Read the model definition and answer for the solid it produces. Units are mm, in the model's axes. A direction names the side the tool comes from. Coordinates: 2 decimals unless noted, no trailing zeros. Write each loop counter-clockwise with the first axis right and the second up, starting at its lowest first coordinate (ties: lowest second). Pieces come first, ordered by that corner, then holes. Notation, with made-up numbers: (29.5, 67) -> (82.5, 67) arc R30 cw to (82.5, 100) -> close; hole circle Ø3 at (32.25, 51). An arc over 180 degrees is marked (long way). One line per item, written item: value. Start each with the question number.
Autodesk Inventor part; units mm, degrees
ref_plane "YZ Plane" through (0, 0, 0) normal (1, 0, 0) x (0, 1, 0)
ref_plane "XZ Plane" through (0, 0, 0) normal (0, 1, 0) x (-1, 0, 0)
ref_plane "XY Plane" through (0, 0, 0) normal (0, 0, 1) x (1, 0, 0)
sketch "Sketch1" plane through (0, 0, 0) normal (0, 1, 0) x (-1, 0, 0)
  circle A0 centre (0, 0) radius 0.465
  dimension "d0" = 0.93
extrude "Extrusion1" add sketch "Sketch1" along normal blind 1.43
sketch "Sketch2" plane through (0, 1.43, 0) normal (0, 1, 0) x (1, 0, 0)
  circle A0 centre (0, 0) radius 0.465
  circle A1 centre (0, 0) radius 0.9625
  line L0 (0, 0) -> (7, 0)
  circle A2 centre (7, 0) radius 0.9625
  line L1 (0, -0.9625) -> (7, -0.9625)
  line L2 (0, 0.9625) -> (7, 0.9625)
  circle A3 centre (7, 0) radius 0.465
  circle A4 centre (5.02, 0) radius 0.465
  circle A5 centre (3.04, 0) radius 0.465
  dimension "d3" = 1.925
  dimension "d4" = 7
  dimension "d5" = 1.925
  dimension "d6" = 0.93
  dimension "d9" = 1.98
extrude "Extrusion2" add sketch "Sketch2" along normal blind 1.43 contours A0 | A1 | A1 L2 A2 L0 A4 A5 | L0 A5 A4 A2 L1 A1 | A2
properties part number "Servo Horn Extension"
1. A cutting plane is placed at C-C on z = 0. Give the vertices of the cut face in (x, y) (1 decimal), then the cut area to 3 significant figures.
2. A cutting plane is placed at D-D on x = 7.25. Give the vertices of the cut face in (y, z).
3. A tool of negligible diameter and unlimited length cuts with its end or side. For faces 4 (the face through (3.47, 2.13, -0.18)), 5 (the face through (0.465, 0.705, -0.02)), from which of +Z, -Z, +X, -X, +Y, -Y can it reach the whole face along a straight path? Write none if from no direction.
4. A cutting plane is placed at A-A on x = 5.02. Give the vertices of the cut face in (y, z) (1 decimal), then the cut area to 3 significant figures.
5. Find the intervals of material crossed by probe 1 along X at (y, z) = (2.15, -0.05); probe 2 along Z at (x, y) = (5.02, 2.05) (1 decimal); probe 3 along Y at (x, z) = (3.5, -0.5), in increasing order. Write a range as from..to.
6. A cutting plane is placed at B-B on y = 2.25. Give the vertices of the cut face in (x, z) (1 decimal).
7. For a pull along Z with two mould halves and no side action, classify faces 1 (the face through (3, 2, 0.962)), 2 (the face through (7.962, 2.135, -0.021)), 3 (the face through (7.43, 2.13, -0.18)) as +Z half, -Z half, draft (parallel to the pull), parting line (faces both ways), or undercut.
8. Given pin 1 (1 mm diameter, centred on x = 5.5, z = -0.5, fed in from -Y), flat-ended and moving along its own axis, determine where the tip first touches the part or whether it passes through.
Derived:
1. outline: (-1, 1.4) -> (-0.5, 1.4) -> (-0.5, 0) -> (0.5, 0) -> (0.5, 1.4) -> (2.6, 1.4) -> (2.6, 2.9) -> (-1, 2.9) -> close; (3.5, 1.4) -> (4.6, 1.4) -> (4.6, 2.9) -> (3.5, 2.9) -> close; (5.5, 1.4) -> (6.5, 1.4) -> (6.5, 2.9) -> (5.5, 2.9) -> close; (7.5, 1.4) -> (8, 1.4) -> (8, 2.9) -> (7.5, 2.9) -> close
1. area: 10.1 mm2
2. outline: (1.43, -0.93) -> (2.86, -0.93) -> (2.86, -0.39) -> (1.43, -0.39) -> close; (1.43, 0.39) -> (2.86, 0.39) -> (2.86, 0.93) -> (1.43, 0.93) -> close
3. face 4: +Y, -Y
3. face 5: -Y
4. outline: (1.4, -1) -> (2.9, -1) -> (2.9, -0.5) -> (1.4, -0.5) -> close; (1.4, 0.5) -> (2.9, 0.5) -> (2.9, 1) -> (1.4, 1) -> close
4. area: 1.42 mm2
5. probe 1: x = -0.96..2.58, 3.5..4.56, 5.48..6.54, 7.46..7.96
5. probe 2: z = -1..-0.5, 0.5..1
5. probe 3: y = 1.43..2.86
6. outline: (0, -1) -> (7, -1) arc R1 ccw to (7, 1) -> (0, 1) arc R1 ccw to start; hole circle Ø0.9 at (3, 0); hole circle Ø0.9 at (5, 0); hole circle Ø0.9 at (7, 0)
7. face 1: +Z half
7. face 2: parting line
7. face 3: undercut
8. pin 1: stops at y = 1.43
